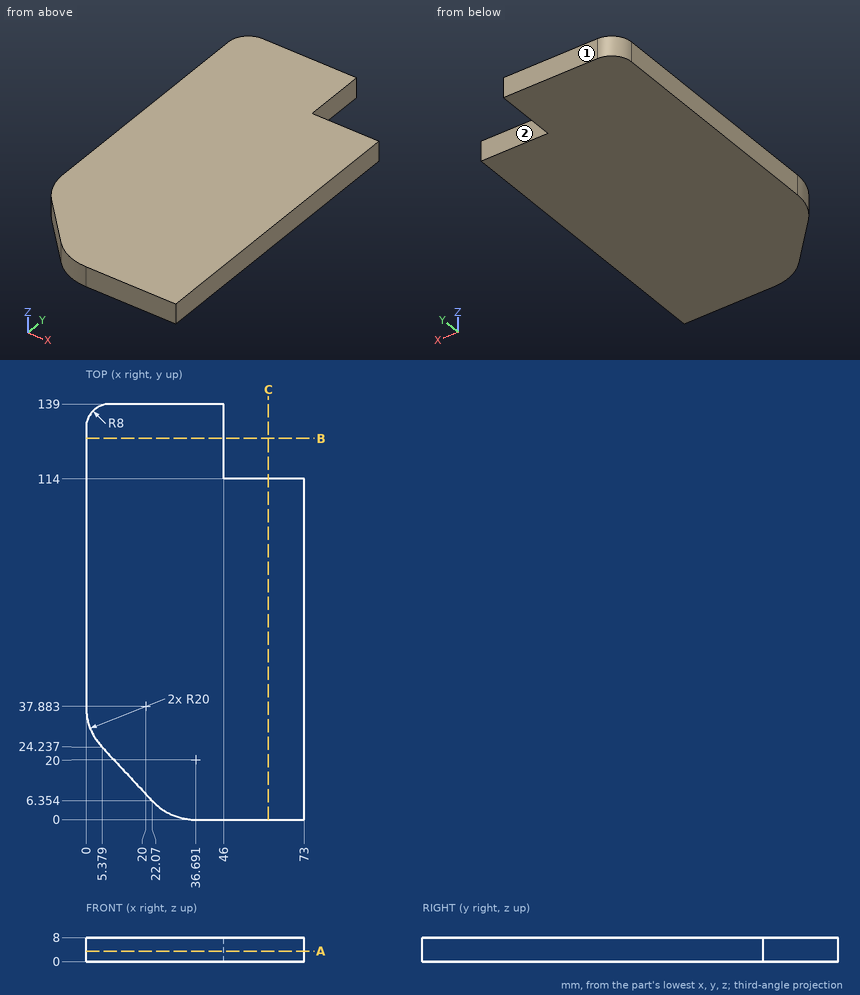
Source: three-view drawing plus pictorial views. Frame: mm from the lowest corner of the part. A direction names the side the tool comes from. Give positions to 0.01 mm unless a question says otherwise; leave off trailing zeros. Order: outer loops, then holes, each group sorted by start corner. A loop starts at its lowest first (then second) coordinate and runs counter-clockwise, first axis right, second up. Notation, with made-up numbers: M 6,-14.75 L 35,-14.75 A30 cw 35,8.25 Z; hole C -7.75,-35 d6. An arc over 180 degrees is marked long. One line per question, with ' | ' between items. Start each with the question number.
1. Section query C-C (x = 61). Return the cut outline in (y, z).
2. Material intervals for probe 1 along Y at (x, z) = (36, 0.75); probe 2 along Y at (x, z) = (69, 7); probe 3 along X at (y, z) = (16.5, 0.75), sorted ascending. Write a range as [from, to].
3. Access query for the marked faces 1 and 2. Directions: +Z, -Z, +X, -X, +Y, -Y. A direction counts if a zero-diameter tool reaches every point of the face in a straight line with its end or side. Return the directions, or none.
4. First-contact query: pin 1 Ø4 at (y, z) = (124.5, 5) entering from +X. Flat tip, straight axial feed; report the tip coordinate or a pass-through.
5. Section query A-A (z = 3.5). Return the cut outline in (x, y), and give its area (3 significant figures).
6. Section query B-B (y = 127.5). Return the cut outline in (x, z), and give its area (3 significant figures).
Here are the results:
1) outline: M 0,0 L 114,0 L 114,8 L 0,8 Z
2) probe 1: [0.01, 139] | probe 2: [0, 114] | probe 3: [12.6, 73]
3) face 1: +Z, -Z, +X, -X, +Y | face 2: +Z, -Z, +X, +Y
4) pin 1: x = 46
5) outline: M 0,37.88 A20 ccw 5.38,24.24 L 22.07,6.35 A20 ccw 36.69,0 L 73,0 L 73,114 L 46,114 L 46,139 L 8,139 A8 ccw 0,131 Z | area: 9,020 mm²
6) outline: M 0,0 L 46,0 L 46,8 L 0,8 Z | area: 368 mm²
